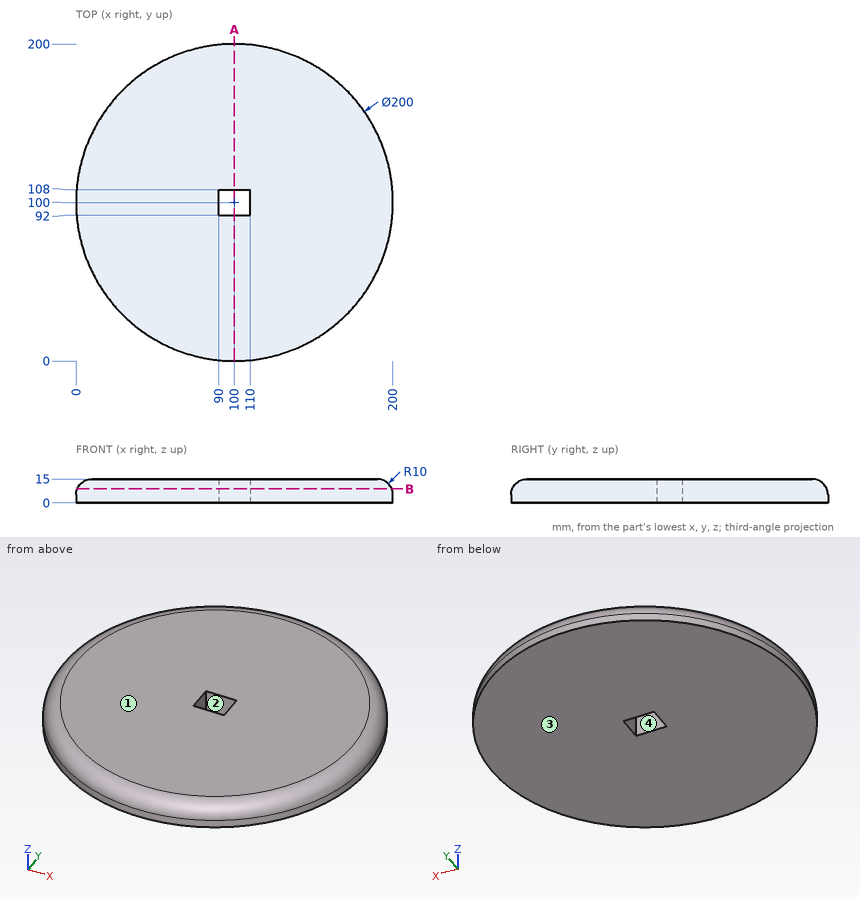
Job drawing, mm, ordinate dimensions from the low corner. One solid piece. A direction names the side the tool comes from. Round coordinates to 2 decimals unless told otherwise and drop trailing zeros. Loops run counter-clockwise (first coordinate to the right, second up) from the corner with the lowest first, then second, coordinate; pieces in that order, holes last.
(1) Drop flat-ended pins along their axis: pin 1 (7.5 mm diameter, centred on x = 96.5, z = 8.5, fed in from -Y); pin 2 (4 mm diameter, centred on y = 37, z = 4.5, fed in from +X); pin 3 (3 mm diameter, centred on x = 41.5, z = 8.5, fed in from -Y). Give the stop position or say it passes through.
(2) Cut at A-A (x = 100). Give the cut face in (y, z).
(3) Wall check: line 1 along X through (y, z) = (38, 1.5); line 2 along Y through (x, z) = (49, 3.75); line 3 along Y through (x, z) = (156.5, 12). Give the ranges that are in metal, low to high.
(4) Cut at B-B (z = 8.75). Give the cut face in (x, y), plus the area to 3 significant figures.
(5) Which spindle directions (+Z, -Z, +X, -X, +Y, -Y) get a long thin tool onto all of the face, cutting with end or side? Do the marked faces 3 and 4. Say none if no direction does.
(6) Two-plate mould, pull along X, no slides. Class the marked faces 1 and 2: +X half, -X half, draft (parallel to the pull), parting line (faces both ways), or undercut.
Findings below:
1. pin 1: stops at y = 0.02
1. pin 2: stops at x = 179.24
1. pin 3: stops at y = 18.44
2. outline: (0, 0) - (92, 0) - (92, 15) - (10, 15) arc R10 ccw to (0, 5) - close; (108, 0) - (200, 0) - (200, 5) arc R10 ccw to (190, 15) - (108, 15) - close
3. line 1: x = 21.54 to 178.46
3. line 2: y = 13.98 to 186.02
3. line 3: y = 20.98 to 179.02
4. outline: circle Ø198.54 at (100, 100); hole (90, 92) - (110, 92) - (110, 108) - (90, 108) - close
4. area: 30,600 mm2
5. face 3: -Z, +X, -X, +Y, -Y
5. face 4: +Z, -Z
6. face 1: draft
6. face 2: undercut
